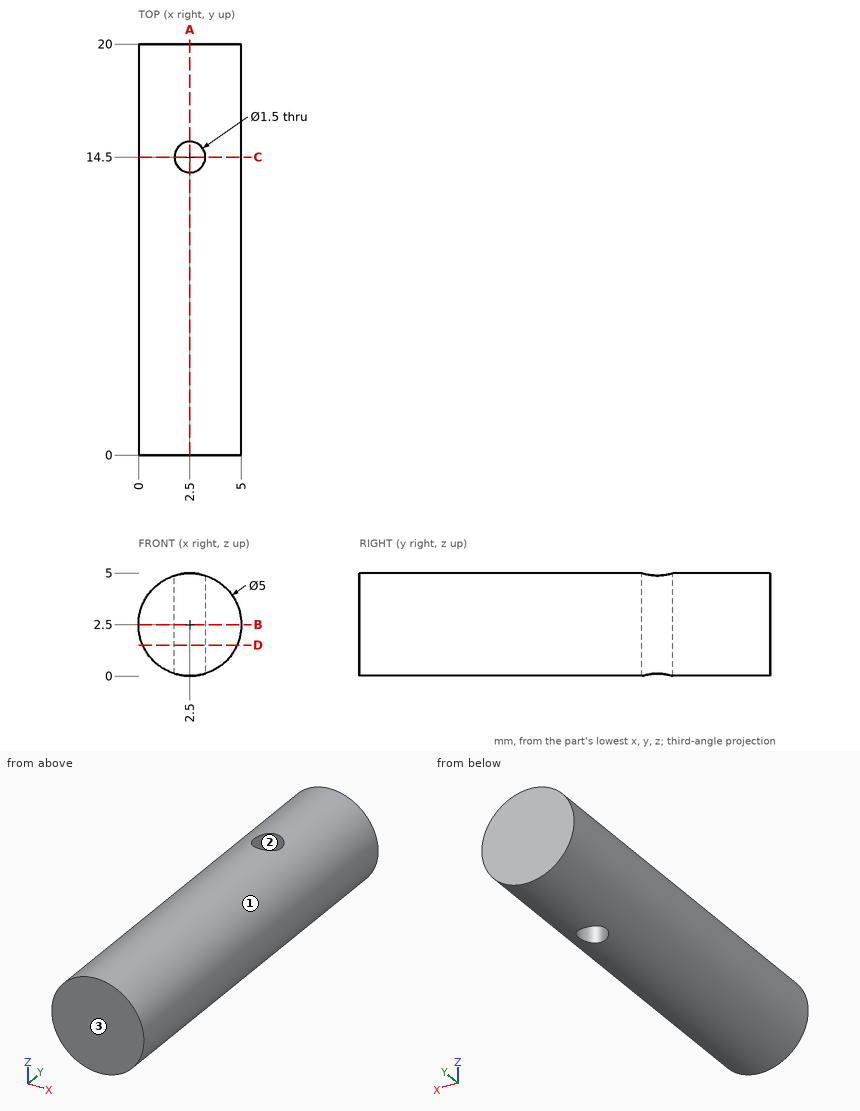
For this review, use the dimensioned drawing (mm, ordinates from the lowest corner) and the shaded views. Give positions to 0.01 mm unless a question says otherwise; leave off trailing zeros. Write each loop counter-clockwise with the first axis right and the second up, starting at its lowest first coordinate (ties: lowest second). Pieces come first, ordered by that corner, then holes. Notation, with made-up numbers: M 62.25,17.5 L 91.25,17.5 A3 ccw 91.25,22.5 Z; hole C -39.75,42 d9. An arc over 180 degrees is marked long. Write item = value, one per line. Start each with the question number.
Q1. We need section D-D (z = 1.5). State the section outline as (x, y) points, plus the area to 3 significant figures.
Q2. We need section C-C (y = 14.5). State the section outline as (x, z) points.
Q3. Mouldability with a two-part tool opening along X and no side actions: class the marked faces 1, 2 and 3 as released by +X, released by -X, zero draft, split by the parting line, or undercut.
Q4. We need section A-A (x = 2.5). State the section outline as (y, z) points, plus the area to 3 significant figures.
Q5. For line 1 (Y direction, x = 2.5, z = 3.3); line 2 (Z direction, x = 2.35, y = 12.5), list the stretches that pass through material, from the lowest coordinate up.
Q6. We need section B-B (z = 2.5). State the section outline as (x, y) points, plus the area to 3 significant figures.
Result set:
q1.outline = M 0.21,0 L 4.79,0 L 4.79,20 L 0.21,20 Z; hole C 2.5,14.5 d1.5
q1.area = 89.9 mm2
q2.outline = M 1.75,0.12 L 1.75,4.88 A2.5 ccw Z; M 3.25,0.12 A2.5 ccw 3.25,4.88 Z
q3.face_1 = split by the parting line
q3.face_2 = undercut
q3.face_3 = zero draft
q4.outline = M 0,0 L 13.75,0 L 13.75,5 L 0,5 Z; M 15.25,0 L 20,0 L 20,5 L 15.25,5 Z
q4.area = 92.5 mm2
q5.line_1 = 0 to 13.75, 15.25 to 20
q5.line_2 = 0 to 5
q6.outline = M 0,0 L 5,0 L 5,20 L 0,20 Z; hole C 2.5,14.5 d1.5
q6.area = 98.2 mm2
